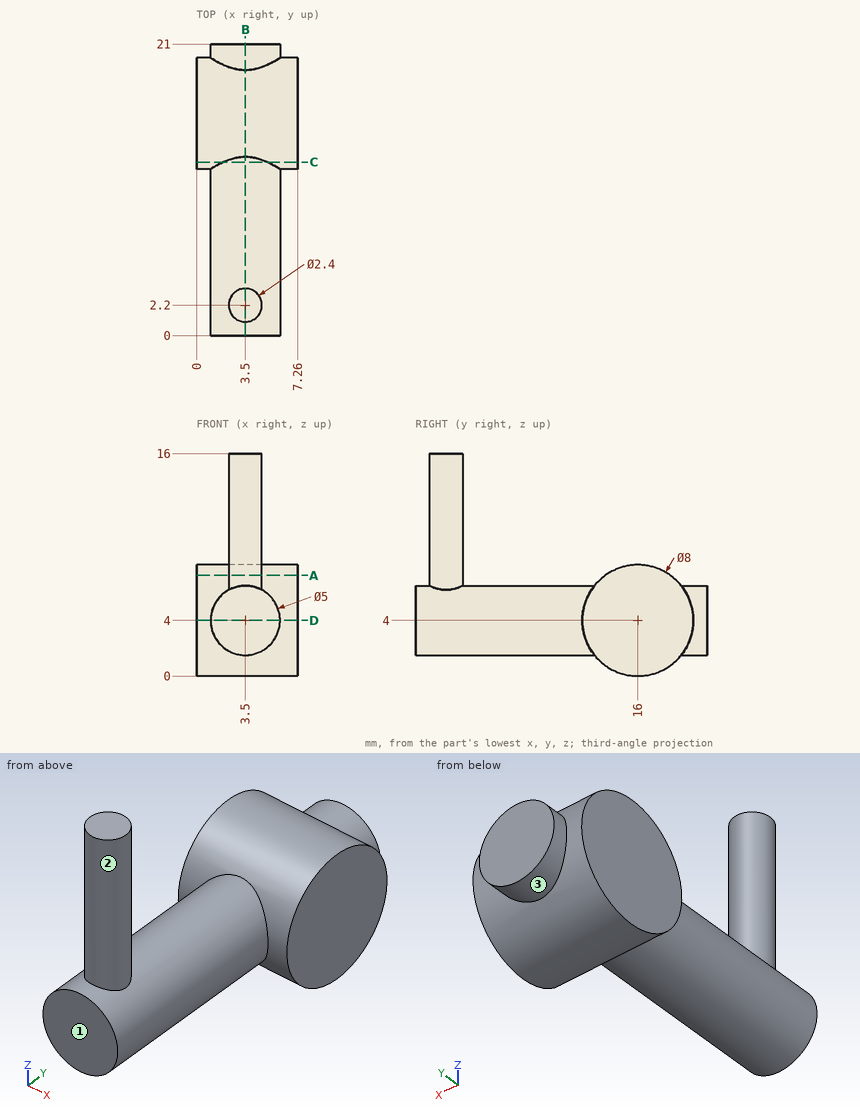
Can you work these out from the drawing? Everything is in mm from the part's minimum corner. A direction names the side the tool comes from. Round coordinates to 2 decimals unless told otherwise and drop trailing zeros. Loops run counter-clockwise (first coordinate to the right, second up) from the corner with the lowest first, then second, coordinate; pieces in that order, holes last. Notation, with made-up numbers: (-9, 18) - (34, 18) arc R3 ccw to (34, 23) - close; hole circle Ø6 at (48, 5). An arc over 180 degrees is marked (long way). One line per question, with ' | ' between items. Start each with the question number.
Q1. For the marked faces 1, 2 and 3, which set-ups out of +Z, -Z, +X, -X, +Y, -Y let a thin tool reach every point of the face, with its end or its side?
Q2. Please list where these lines run through material, in increasing order: line 1 (Y direction, x = 1.5, z = 6.5); line 2 (Y direction, x = 3.25, z = 10.75); line 3 (Z direction, x = 1.25, y = 4). Write a range as [from, to].
Q3. Will these pins go through, and if not, where does the flat tip stop? pin 1 (4 mm diameter, centred on y = 3.5, z = 12, fed in from -X); pin 2 (4 mm diameter, centred on x = 6, y = 10, fed in from +Z).
Q4. I want a section at B-B (x = 3.5). Write out the boundary of the cut face in (y, z), then the cut area to 3 significant figures.
Q5. I want a section at D-D (z = 4). Write out the boundary of the cut face in (x, y), then the cut area to 3 significant figures.
Q6. I want a section at A-A (z = 7.25). Write out the boundary of the cut face in (x, y).
Q7. I want a section at C-C (y = 12.5). Write out the boundary of the cut face in (x, z).
Response values:
1) face 1: +Z, -Z, +X, -X, -Y | face 2: +Z | face 3: +Y
2) line 1: y = [12.88, 19.12] | line 2: y = [1.03, 3.37] | line 3: z = [2.91, 5.09]
3) pin 1: stops at x = 2.3 | pin 2: stops at z = 6.45
4) outline: (0, 1.5) - (12.88, 1.5) arc R4 ccw to (19.12, 1.5) - (21, 1.5) - (21, 6.5) - (19.12, 6.5) arc R4 ccw to (12.88, 6.5) - (3.4, 6.5) - (3.4, 16) - (1, 16) - (1, 6.5) - (0, 6.5) - close | area: 141 mm²
5) outline: (0, 12) - (1, 12) - (1, 0) - (6, 0) - (6, 12) - (7.26, 12) - (7.26, 20) - (6, 20) - (6, 21) - (1, 21) - (1, 20) - (0, 20) - close | area: 123 mm²
6) outline: (0, 13.67) - (7.26, 13.67) - (7.26, 18.33) - (0, 18.33) - close; circle Ø2.4 at (3.5, 2.2)
7) outline: (0, 2.06) - (1.92, 2.06) arc R2.5 ccw to (5.08, 2.06) - (7.26, 2.06) - (7.26, 5.94) - (5.08, 5.94) arc R2.5 ccw to (1.92, 5.94) - (0, 5.94) - close
